Work out the finished part from the listing and answer in its coordinate system (mm). Coordinates: 2 decimals unless noted, no trailing zeros. Loops run counter-clockwise (first coordinate to the right, second up) from the corner with the lowest first, then second, coordinate; pieces in that order, holes last. Notation, with made-up numbers: (-29, 70.5) -> (-20, 70.5) arc R24 cw to (-20, 98.5) -> close; hole circle Ø7 at (60.5, 57). An arc over 180 degrees is marked (long way). One line per question, with ' | ' between items.
```python
from build123d import *

# Parameters (mm, degrees)
F0_R     = 10.795
F1_DEPTH = 1.524


with BuildPart() as f1:
    # F0 (on Front) → F1 (new body)
    with BuildSketch(Plane.XZ):
        with BuildLine():
            ThreePointArc((-4.439889, 25.008946), (16.315435, 19.467064), (25.4, 0))
            ThreePointArc((25.4, 0), (23.451217, -9.75707), (17.903904, -18.016943))
            Line((17.903904, -18.016943), (42.672, 6.595757))
            ThreePointArc((42.672, 6.595757), (50.317232, 11.678079), (59.32263, 13.462))
            Line((59.32263, 13.462), (152.913683, 13.462))
            ThreePointArc((152.913683, 13.462), (162.418002, 16.215479), (168.97857, 23.623089))
            Line((168.97857, 23.623089), (169.305095, 24.311584))
            ThreePointArc((169.305095, 24.311584), (169.156757, 26.75776), (167.010111, 27.94))
            Line((167.010111, 27.94), (12.070111, 27.94))
            Line((12.070111, 27.94), (-4.439889, 25.008946))
        make_face()
        with BuildLine():
            ThreePointArc((17.903904, -18.016943), (23.451217, -9.75707), (25.4, 0))
            ThreePointArc((25.4, 0), (16.315435, 19.467064), (-4.439889, 25.008946))
            ThreePointArc((-4.439889, 25.008946), (-22.541666, -11.706122), (17.903904, -18.016943))
        make_face()
        Circle(F0_R, mode=Mode.SUBTRACT)
    extrude(amount=F1_DEPTH)


solid = f1.part
```
1) Find section A-A (y = -1.1). Write down the section's boundary in (x, z) (3 decimals).
Check values:
outline: (-4.44, 25.009) arc R25.4 ccw (long way) to (17.904, -18.017) -> (42.672, 6.596) arc R23.622 cw to (59.323, 13.462) -> (152.914, 13.462) arc R17.78 ccw to (168.979, 23.623) -> (169.305, 24.312) arc R2.54 ccw to (167.01, 27.94) -> (12.07, 27.94) -> close; hole circle Ø21.59 at (0, 0)
2) Flat-ended cylindrical pins translate along their axes: pin 1 (2 mm diameter, centred on x = -4.5, z = 11, fed in from +Y); pin 2 (3 mm diameter, centred on x = 79, z = 11, fed in from +Y). Find the tip coordinate at first contact, or state that the pin passes through.
Check values:
pin 1: stops at y = 0 | pin 2: passes through
3) Find section D-D (x = 131). Write down the section's boundary in (y, z), plus the area to 3 significant figures.
Check values:
outline: (-1.52, 13.46) -> (0, 13.46) -> (0, 27.94) -> (-1.52, 27.94) -> close | area: 22.1 mm^2
4) Find section C-C (z = 0). Write down the section's boundary in (x, y) (3 decimals).
Check values:
outline: (-25.4, -1.524) -> (-10.795, -1.524) -> (-10.795, 0) -> (-25.4, 0) -> close; (10.795, -1.524) -> (36.035, -1.524) -> (36.035, 0) -> (10.795, 0) -> close
5) The mould has two halves that part along X. Classify faces 1 (the face through (-7.956, -0.751, 7.296)), 2 (the face through (-22.84, -0.75, -11.11)), 3 (the face through (162.3, -0.75, 16.14)): released by +X, released by -X, zero draft, split by the parting line, or undercut.
Check values:
face 1: undercut | face 2: split by the parting line | face 3: released by +X
6) Find section B-B (x = 0). Write down the section's boundary in (y, z) (3 decimals).
Check values:
outline: (-1.524, -25.4) -> (0, -25.4) -> (0, -10.795) -> (-1.524, -10.795) -> close; (-1.524, 10.795) -> (0, 10.795) -> (0, 25.797) -> (-1.524, 25.797) -> close
7) Find the intervals of material crossed by line 1 along Z through (x, y) = (0, -1.2) (3 decimals); line 2 along Z through (x, y) = (90, -0.1); line 3 along X through (y, z) = (-1.35, -3), in increasing order.
Check values:
line 1: z = -25.4 to -10.795, 10.795 to 25.797 | line 2: z = 13.46 to 27.94 | line 3: x = -25.22 to -10.37, 10.37 to 33.02
